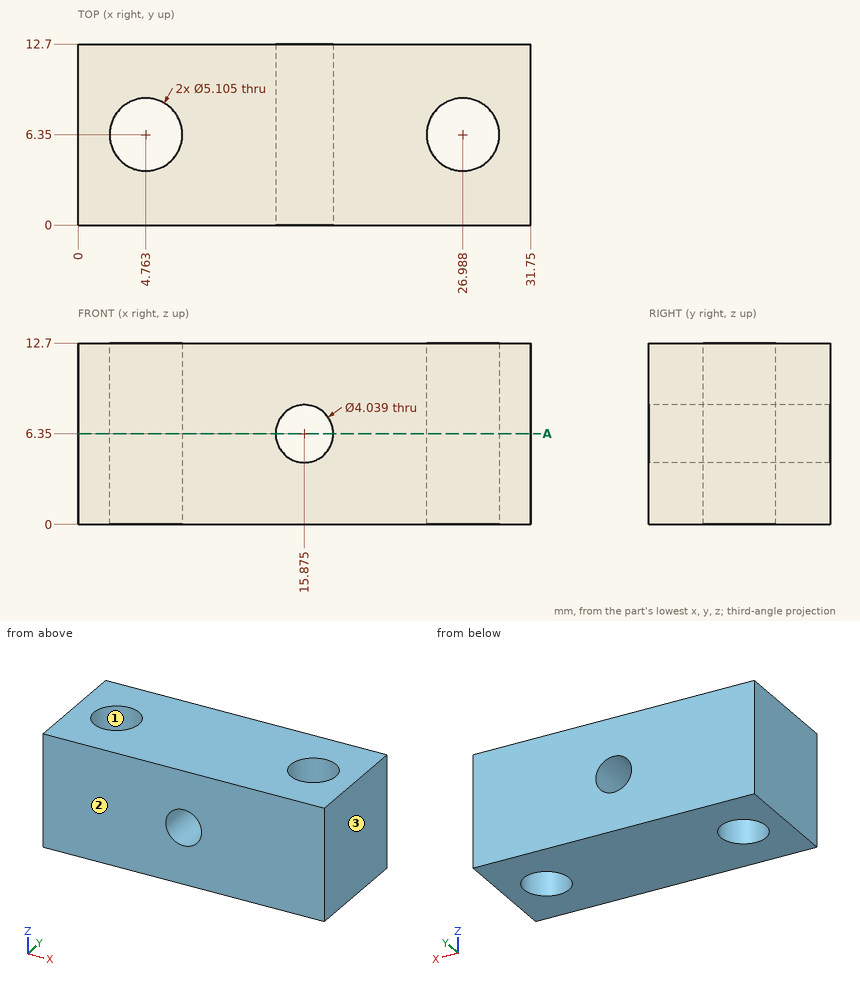
Verification items for this drawing (mm, ordinates from the low corner). Coordinates: 2 decimals unless noted, no trailing zeros. Write each question's results on one line, items separated by ' | '.
1) Scan lines: line 1 along X through (y, z) = (3, 6.5); line 2 along Y through (x, z) = (5, 9.5); line 3 along Y through (x, z) = (7, 7) (1 decimal). Record each from-to range of solid material in increasing order. Write a range as [from, to].
Solved:
line 1: x = [0, 13.86], [17.89, 31.75] | line 2: y = [0, 3.81], [8.89, 12.7] | line 3: y = [0, 5.1], [7.6, 12.7]
2) Section check A-A on z = 6.35. Give the number of separate pieces and of enclosed holes in the cut face, plus the area to 3 significant figures.
Solved:
separate pieces: 2 | enclosed holes: 2 | area: 311 mm²
3) Release check for a two-part mould opening along X. For the marked faces 1, 2 and 3 record: pulls with the +X half, pulls with the -X half, needs draft (parallel to the pull), parting line crosses it, or undercut.
Solved:
face 1: undercut | face 2: needs draft | face 3: pulls with the +X half
4) Gauge pin test, flat end, axial feed: pin 1 Ø4 at (y, z) = (2.5, 8.5) entering from -X. Record the tip position at first contact, or that the pin passes through.
Solved:
pin 1: stops at x = 0
